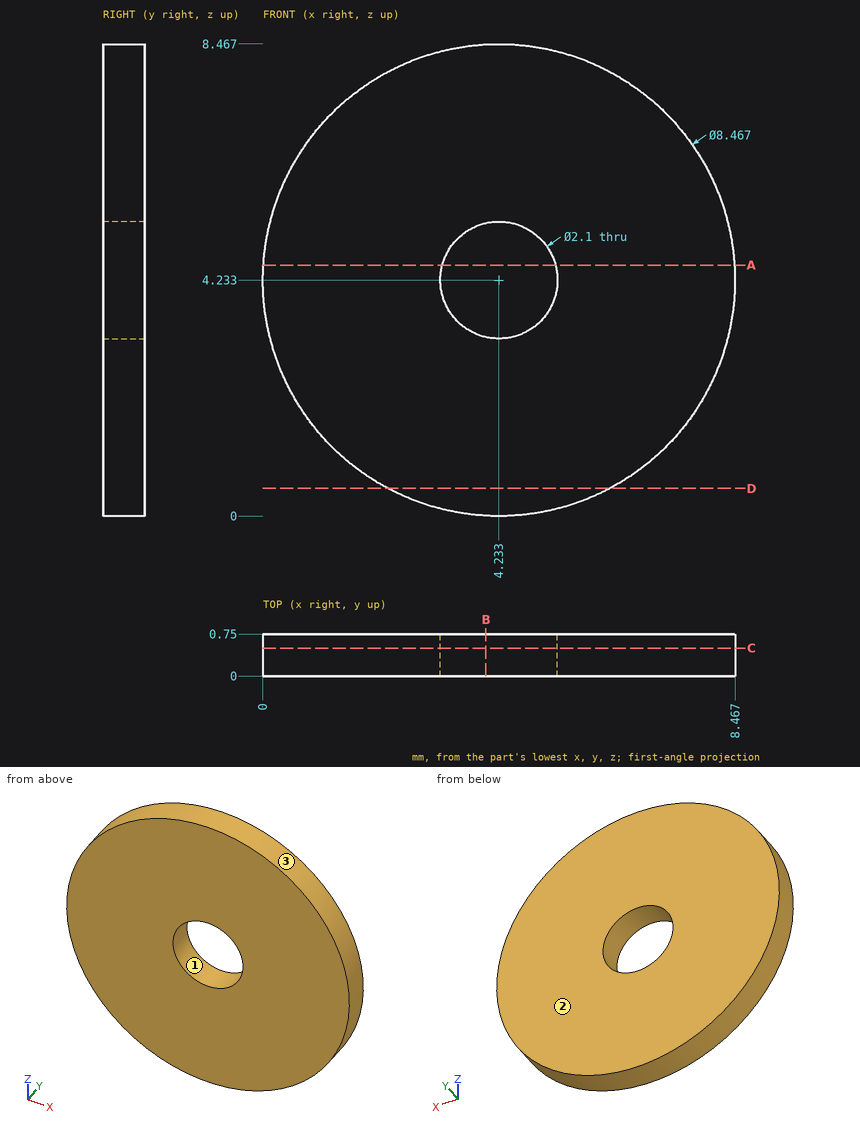
Job drawing, mm, ordinate dimensions from the low corner. One solid piece. Give positions to 0.01 mm unless a question says otherwise; leave off trailing zeros. Loops run counter-clockwise (first coordinate to the right, second up) from the corner with the lowest first, then second, coordinate; pieces in that order, holes last. Notation, with made-up numbers: M -26,-18.75 L -22,-18.75 A28 cw -22,2.25 Z; hole C -10,3.25 d1. An arc over 180 degrees is marked long. Return JSON: item names as keys, results as strings.
1) Saw through at D-D, the plane z = 0.5. List the corners of the cut face in (x, y).
Calculated:
{"outline": "M 2.24,0 L 6.23,0 L 6.23,0.75 L 2.24,0.75 Z"}
2) Saw through at B-B, the plane x = 4. List the corners of the cut face in (y, z).
Calculated:
{"outline": "M 0,0.01 L 0.75,0.01 L 0.75,3.21 L 0,3.21 Z; M 0,5.26 L 0.75,5.26 L 0.75,8.46 L 0,8.46 Z"}
3) Saw through at A-A, the plane z = 4.5. List the corners of the cut face in (x, y).
Calculated:
{"outline": "M 0.01,0 L 3.22,0 L 3.22,0.75 L 0.01,0.75 Z; M 5.25,0 L 8.46,0 L 8.46,0.75 L 5.25,0.75 Z"}
4) Pull direction X, two halves, no side cores. Call the marked faces 1, 2 and 3: released by +X, released by -X, zero draft, split by the parting line, or undercut.
Calculated:
{"face 1": "undercut", "face 2": "zero draft", "face 3": "split by the parting line"}
5) Drill centre lines: line 1 (Z direction, x = 4.25, y = 0.15); line 2 (Z direction, x = 3.75, y = 0.25) (1 decimal). Where is each one in solid material? Low to high.
Calculated:
{"line 1": "z = 0 to 3.18, 5.28 to 8.47", "line 2": "z = 0 to 3.3, 5.2 to 8.4"}
6) Saw through at C-C, the plane y = 0.5. List the corners of the cut face in (x, z).
Calculated:
{"outline": "C 4.23,4.23 d8.47; hole C 4.23,4.23 d2.1"}
